Verification items for the finished model (mm, model axes). Face numbers are marked on the shaded views. A direction names the side the tool comes from. Round coordinates to 2 decimals unless told otherwise and drop trailing zeros. Order: outer loops, then holes, each group sorted by start corner. A loop starts at its lowest first (then second) coordinate and runs counter-clockwise, first axis right, second up. Notation, with made-up numbers: (27.25, 1) -> (56.25, 1) arc R34 ccw to (56.25, 38) -> close; hole circle Ø4 at (70.25, 32). An arc over 180 degrees is marked (long way). Answer in a Markdown table with one row per item. Add a question column.
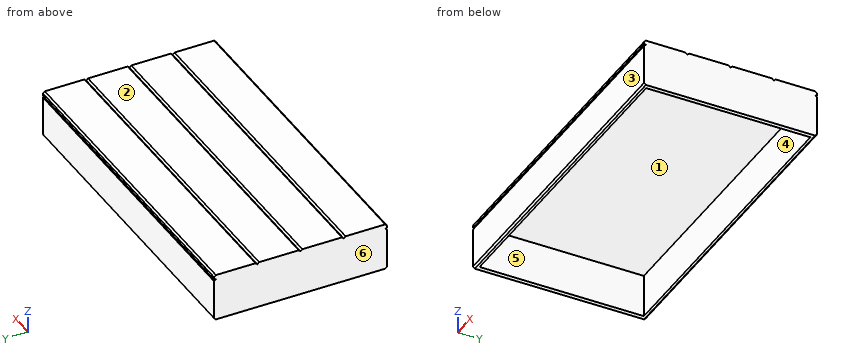
```python
from build123d import *

# Parameters (mm, degrees)
F0_W      = 900
F0_H      = 480
F1_DEPTH  = 12
F3_DEPTH  = 900.001
F4_W      = 900
F4_H      = 12
F5_DEPTH  = 120
F6_W      = 900
F6_H      = 12
F7_DEPTH  = 120
F8_W      = 12
F8_H      = 456
F9_DEPTH  = 120
F10_W     = 12
F10_H     = 456
F11_DEPTH = 120
F13_DEPTH = 900.001
F15_DEPTH = 900.001


with BuildPart() as f1:
    # F0 (on Top) → F1 (new body)
    with BuildSketch(Plane.XY):
        with Locations((393.5734190047, 233.7786073424)):
            Rectangle(F0_W, F0_H)
    extrude(amount=F1_DEPTH)

    # F2 (on face) → F3 (cut, through all)
    with BuildSketch(Plane.YZ.offset(843.5734190047)):
        Polygon((-1.2213926576, 12), (-6.2213926576, 12), (-6.2213926576, 7), align=None)
        Polygon((118.7786073424, 12), (113.7786073424, 12), (108.7786073424, 12), (113.7786073424, 7), align=None)
        Polygon((238.7786073424, 12), (233.7786073424, 12), (228.7786073424, 12), (233.7786073424, 7), align=None)
        Polygon((358.7786073424, 12), (353.7786073424, 12), (348.7786073424, 12), (353.7786073424, 7), align=None)
        Polygon((473.7786073424, 7), (473.7786073424, 12), (468.7786073424, 12), align=None)
    extrude(amount=-F3_DEPTH, mode=Mode.SUBTRACT)

    # F4 (on face) → F5 (join)
    with BuildSketch(Plane(origin=(0, 0, 0), x_dir=(1, 0, 0), z_dir=(0, 0, -1))):
        with Locations((393.5734190047, -467.7786073424)):
            Rectangle(F4_W, F4_H)
    extrude(amount=F5_DEPTH)

    # F6 (on face) → F7 (join)
    with BuildSketch(Plane(origin=(0, 0, 0), x_dir=(1, 0, 0), z_dir=(0, 0, -1))):
        with Locations((393.5734190047, 0.2213926576)):
            Rectangle(F6_W, F6_H)
    extrude(amount=F7_DEPTH)

    # F8 (on face) → F9 (join)
    with BuildSketch(Plane(origin=(0, 0, 0), x_dir=(1, 0, 0), z_dir=(0, 0, -1))):
        with Locations((-50.4265809953, -233.7786073424)):
            Rectangle(F8_W, F8_H)
    extrude(amount=F9_DEPTH)

    # F10 (on face) → F11 (join)
    with BuildSketch(Plane(origin=(0, 0, 0), x_dir=(1, 0, 0), z_dir=(0, 0, -1))):
        with Locations((837.5734190047, -233.7786073424)):
            Rectangle(F10_W, F10_H)
    extrude(amount=F11_DEPTH)

    # F12 (on face) → F13 (cut, through all)
    with BuildSketch(Plane.YZ.offset(843.5734190047)):
        Polygon((-1.2213926576, 0), (-6.2213926576, 0), (-6.2213926576, -5), align=None)
        Polygon((-6.2213926576, -115), (-6.2213926576, -120), (-1.2213926576, -120), align=None)
    extrude(amount=-F13_DEPTH, mode=Mode.SUBTRACT)

    # F14 (on face) → F15 (cut, through all)
    with BuildSketch(Plane(origin=(-56.4265809953, 0, 0), x_dir=(0, -1, 0), z_dir=(-1, 0, 0))):
        Polygon((-468.7786073424, 0), (-473.7786073424, 0), (-473.7786073424, -5), align=None)
        Polygon((-473.7786073424, -115), (-473.7786073424, -120), (-468.7786073424, -120), align=None)
    extrude(amount=-F15_DEPTH, mode=Mode.SUBTRACT)


solid = f1.part
```
1) Cross-section at A-A, the plane z = -28. Record the boundary of the cut face in (x, y), and give its area (3 significant figures).
2) Tool access check on the marked faces 1 and 2. Record the directions out of +Z, -Z, +X, -X, +Y, -Y that give a thin tool (end or side, any length) a straight path to the whole face; none if there is none.
3) Draft check along X on the marked faces 3, 4, 5 and 6. Enter one of: +X half, -X half, draft (parallel to the pull), parting line (faces both ways), or undercut.
4) Cross-section at C-C, the plane y = 252.5. Record the boundary of the cut face in (x, z).
5) Cross-section at B-B, the plane x = 237.5. Record the boundary of the cut face in (y, z), and give its area (3 significant figures).
6) Depth check by flat-ended pin: P1, Ø1, axis at x = 367, y = 248, coming from the -Z side; P2, Ø4, axis at x = 509.5, y = 471, coming from the -Z side; P3, Ø4, axis at x = 416.5, y = -4.5, coming from the -Z side. Enter the tip coordinate at first touch or a pass-through.
7) Thickness scan on L1, parallel to Y at x = 172, z = -97.5; L2, parallel to X at y = 118, z = -89; L3, parallel to Z at x = 123, y = 437. Record the ranges inside material, lowest first. Write a range as [from, to].
Results below:
| question | item | result |
|---|---|---|
| 1 | outline | (-56.43, -6.22) -> (843.57, -6.22) -> (843.57, 473.78) -> (-56.43, 473.78) -> close; hole (-44.43, 5.78) -> (831.57, 5.78) -> (831.57, 461.78) -> (-44.43, 461.78) -> close |
| 1 | area | 32,500 mm² |
| 2 | face 1 | -Z |
| 2 | face 2 | +Z, +X, -X, +Y, -Y |
| 3 | face 3 | draft |
| 3 | face 4 | undercut |
| 3 | face 5 | undercut |
| 3 | face 6 | -X half |
| 4 | outline | (-56.43, -120) -> (-44.43, -120) -> (-44.43, 0) -> (831.57, 0) -> (831.57, -120) -> (843.57, -120) -> (843.57, 12) -> (-56.43, 12) -> close |
| 5 | outline | (-6.22, -115) -> (-1.22, -120) -> (5.78, -120) -> (5.78, 0) -> (461.78, 0) -> (461.78, -120) -> (468.78, -120) -> (473.78, -115) -> (473.78, -5) -> (468.78, 0) -> (473.78, 0) -> (473.78, 7) -> (468.78, 12) -> (358.78, 12) -> (353.78, 7) -> (348.78, 12) -> (238.78, 12) -> (233.78, 7) -> (228.78, 12) -> (118.78, 12) -> (113.78, 7) -> (108.78, 12) -> (-1.22, 12) -> (-6.22, 7) -> (-6.22, 0) -> (-1.22, 0) -> (-6.22, -5) -> close |
| 5 | area | 8,490 mm² |
| 6 | P1 | z = 0 |
| 6 | P2 | z = -119.78 |
| 6 | P3 | z = -118.72 |
| 7 | L1 | [-6.22, 5.78], [461.78, 473.78] |
| 7 | L2 | [-56.43, -44.43], [831.57, 843.57] |
| 7 | L3 | [0, 12] |
